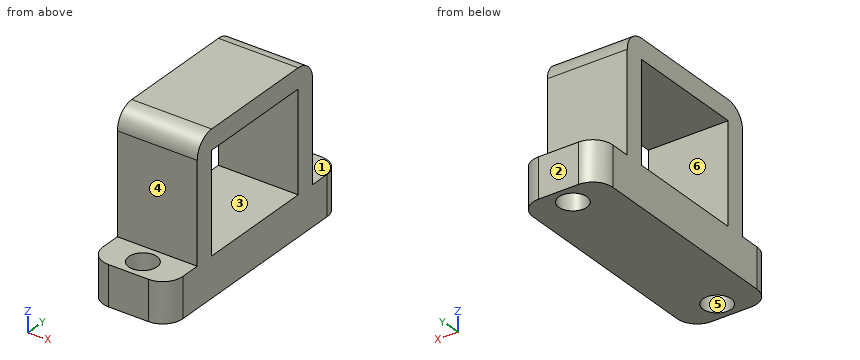
Autodesk Inventor part; units mm, degrees
ref_plane "YZ Plane" through (0, 0, 0) normal (1, 0, 0) x (0, 1, 0)
ref_plane "XZ Plane" through (0, 0, 0) normal (0, 1, 0) x (-1, 0, 0)
ref_plane "XY Plane" through (0, 0, 0) normal (0, 0, 1) x (1, 0, 0)
sketch "Sketch1" plane through (0, 0, 0) normal (0, 0, 1) x (1, 0, 0)
  line L0 (6.35, -12.7) -> (-6.35, -12.7)
  line L1 (-6.35, -12.7) -> (-6.35, 12.7)
  line L2 (-6.35, 12.7) -> (6.35, 12.7)
  line L3 (6.35, 12.7) -> (6.35, -12.7)
  line L4 (6.35, -12.7) -> (-6.35, 12.7) construction
  line L5 (-6.35, -12.7) -> (6.35, 12.7) construction
  line L6 (-6.35, 12.7) -> (6.35, 12.7)
  line L7 (6.35, 12.7) -> (6.35, 19.05)
  line L8 (6.35, 19.05) -> (-6.35, 19.05)
  line L9 (-6.35, 19.05) -> (-6.35, 12.7)
  line L10 (-6.35, -12.7) -> (6.35, -12.7)
  line L11 (6.35, -12.7) -> (6.35, -19.05)
  line L12 (6.35, -19.05) -> (-6.35, -19.05)
  line L13 (-6.35, -19.05) -> (-6.35, -12.7)
  circle A0 centre (0, 15.875) radius 2.25
  circle A1 centre (0, -15.875) radius 2.25
  point P0 (0, 0)
  dimension "d0" = 12.7
  dimension "d1" = 25.4
  dimension "d2" = 6.35
  dimension "d3" = 6.35
  dimension "d4" = 4.5
  dimension "d5" = 4.5
extrude "Extrusion1" add sketch "Sketch1" along normal blind 6.35 contours L11 L12 L13 L0 | L2 L9 L8 L7
extrude "Extrusion2" add sketch "Sketch1" along normal blind 25.4 contours L0 L1 L2 L3
sketch "Sketch2" plane through (6.35, -19.05, 0) normal (1, 0, 0) x (0, 0, -1)
  line L0 (0, 0) -> (0, 38.1)
  line L1 (0, 38.1) -> (-6.35, 38.1)
  line L2 (-6.35, 31.75) -> (-6.35, 38.1)
  line L3 (-6.35, 31.75) -> (-25.4, 31.75)
  line L4 (-25.4, 6.35) -> (-25.4, 31.75)
  line L5 (-6.35, 6.35) -> (-25.4, 6.35)
  line L6 (-6.35, 0) -> (-6.35, 6.35)
  line L7 (0, 0) -> (-6.35, 0)
  line L8 (-6.35, 38.1) -> (-6.35, 31.75)
  line L9 (-6.35, 6.35) -> (-6.35, 0)
  line L10 (-6.35, 31.75) -> (-6.35, 6.35)
  line L11 (-6.35, 28.575) -> (-22.225, 28.575)
  line L12 (-22.225, 28.575) -> (-22.225, 9.525)
  line L13 (-22.225, 9.525) -> (-6.35, 9.525)
  point P0 (0, 19.05)
  dimension "d10" = 3.175
extrude "Extrusion3" cut sketch "Sketch2" against normal through all contours L13 L12 L11 L10
fillet "Fillet1" radius 3.175 6 edges at (-6.35, 19.05, 3.175) (6.35, 19.05, 3.175) (0, 12.7, 25.4) (0, -12.7, 25.4) (6.35, -19.05, 3.175) (-6.35, -19.05, 3.175)
properties part number "Latch_For_Climb_And_Drone"
Part model, mm, in its own coordinate system. Face numbers are marked on the shaded views. A direction names the side the tool comes from. Give positions to 0.01 mm unless a question says otherwise; leave off trailing zeros. Loops run counter-clockwise (first coordinate to the right, second up) from the corner with the lowest first, then second, coordinate; pieces in that order, holes last. Notation, with made-up numbers: (80, -28.5) -> (134, -28.5) arc R23 cw to (134, -8.5) -> close; hole circle Ø10 at (16.25, -5). An arc over 180 degrees is marked (long way). Write each question's results on one line, items separated by ' | '. Start each with the question number.
Q1. Band-saw the part on D-D on z = 3. List the corners of the cut face in (x, y) (3 decimals), plus the area to 3 significant figures.
Q2. Wall check: L1, parallel to Y at x = 0, z = 2 (3 decimals); L2, parallel to Y at x = -5, z = 21 (3 decimals); L3, parallel to Z at x = -1.5, y = -5.5 (3 decimals). Give the ranges that are in metal, low to high.
Q3. Which spindle directions (+Z, -Z, +X, -X, +Y, -Y) get a long thin tool onto all of the face, cutting with end or side? Do the marked faces 4, 5 and 6. Say none if no direction does.
Q4. Band-saw the part on A-A on x = 0. List the corners of the cut face in (y, z) (3 decimals).
Q5. Pin check, flat tips, straight feed: P1, Ø6, axis at x = 0, y = -15.875, coming from the +Z side; P2, Ø6, axis at x = 0, y = 15.875, coming from the -Z side; P3, Ø4, axis at x = -2, z = 11.5, coming from the +Y side. Stop position of each tip, or through.
Q6. Band-saw the part on C-C on y = -1. List the corners of the cut face in (x, z) (3 decimals), plus the area to 3 significant figures.
Q7. Band-saw the part on B-B on z = 21.75. List the corners of the cut face in (x, y) (3 decimals).
Q8. Pull direction Z, two halves, no side cores. Call the marked faces 1, 2 and 3: +Z half, -Z half, draft (parallel to the pull), parting line (faces both ways), or undercut.
Results are:
1) outline: (-6.35, -15.875) arc R3.175 ccw to (-3.175, -19.05) -> (3.175, -19.05) arc R3.175 ccw to (6.35, -15.875) -> (6.35, 15.875) arc R3.175 ccw to (3.175, 19.05) -> (-3.175, 19.05) arc R3.175 ccw to (-6.35, 15.875) -> close; hole circle Ø4.5 at (0, -15.875); hole circle Ø4.5 at (0, 15.875) | area: 443 mm²
2) L1: y = -19.05 to -18.125, -13.625 to 13.625, 18.125 to 19.05 | L2: y = -12.7 to -9.525, 9.525 to 12.7 | L3: z = 0 to 6.35, 22.225 to 25.4
3) face 4: +Z, +X, -X, -Y | face 5: +Z, -Z | face 6: +X, -X
4) outline: (-19.05, 0) -> (-18.125, 0) -> (-18.125, 6.35) -> (-19.05, 6.35) -> close; (-13.625, 0) -> (13.625, 0) -> (13.625, 6.35) -> (12.7, 6.35) -> (12.7, 22.225) arc R3.175 ccw to (9.525, 25.4) -> (-9.525, 25.4) arc R3.175 ccw to (-12.7, 22.225) -> (-12.7, 6.35) -> (-13.625, 6.35) -> close; (18.125, 0) -> (19.05, 0) -> (19.05, 6.35) -> (18.125, 6.35) -> close; hole (-9.525, 6.35) -> (9.525, 6.35) -> (9.525, 22.225) -> (-9.525, 22.225) -> close
5) P1: stops at z = 6.35 | P2: stops at z = 0 | P3: stops at y = 12.7
6) outline: (-6.35, 0) -> (6.35, 0) -> (6.35, 6.35) -> (-6.35, 6.35) -> close; (-6.35, 22.225) -> (6.35, 22.225) -> (6.35, 25.4) -> (-6.35, 25.4) -> close | area: 121 mm²
7) outline: (-6.35, -12.7) -> (6.35, -12.7) -> (6.35, -9.525) -> (-6.35, -9.525) -> close; (-6.35, 9.525) -> (6.35, 9.525) -> (6.35, 12.7) -> (-6.35, 12.7) -> close
8) face 1: +Z half | face 2: draft | face 3: undercut
